Source: three-view drawing plus pictorial views. Frame: mm from the lowest corner of the part. Give positions to 0.01 mm unless a question says otherwise; leave off trailing zeros. Loops run counter-clockwise (first coordinate to the right, second up) from the corner with the lowest first, then second, coordinate; pieces in that order, holes last. Notation, with made-up numbers: (-8.75, 68.25) -> (25.25, 68.25) arc R18 ccw to (25.25, 90.25) -> close; hole circle Ø5 at (37, -26.75). An arc over 180 degrees is marked (long way). One line per item, written item: value. Start each with the question number.
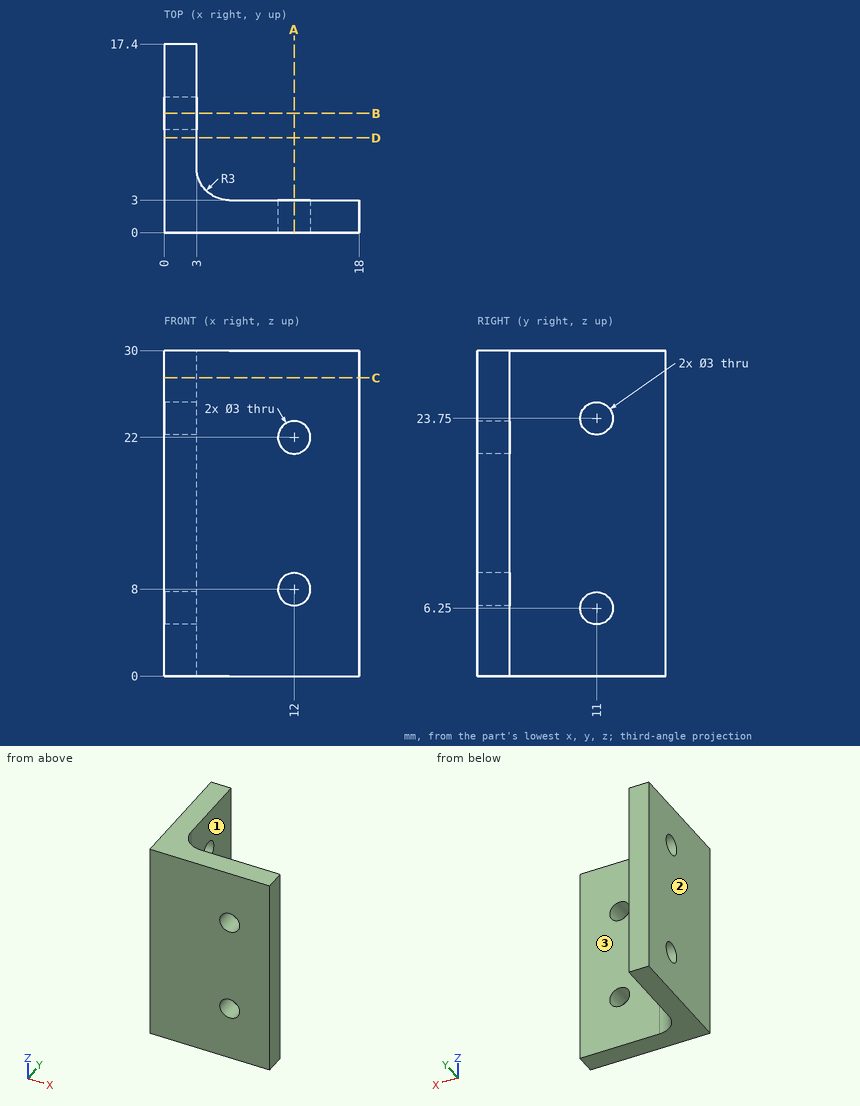
Item 1: Section A-A, the plane x = 12. Output: boundary loops of the cut face in (y, z), then the cut area to 3 significant figures.
Item 2: Ray query, line 1 along Z through (x, y) = (1, 11); line 2 along Y through (x, z) = (2.45, 23.75); line 3 along X through (y, z) = (2.35, 8). Return the intervals inside material, ascending. Write a range as [from, to].
Item 3: Pin query (flat end, axial travel): pin 1 (10 mm diameter, centred on y = 15.5, z = 23, fed in from +X); pin 2 (5 mm diameter, centred on x = 11, z = 18.5, fed in from +Y). Return the tip coordinate at first contact, or that it passes through.
Item 4: Section B-B, the plane y = 11. Output: boundary loops of the cut face in (x, z).
Item 5: Section C-C, the plane z = 27.5. Output: boundary loops of the cut face in (x, y), then the cut area to 3 significant figures.
Item 6: Mould query, pull axis X, two halves, no side actions, for the marked faces 1, 2 and 3. Classes: pulls with the +X half, pulls with the -X half, needs draft (parallel to the pull), parting line crosses it, or undercut.
Item 7: Section D-D, the plane y = 8.75. Output: boundary loops of the cut face in (x, z).
Geometry check:
1. outline: (0, 0) -> (3, 0) -> (3, 6.5) -> (0, 6.5) -> close; (0, 9.5) -> (3, 9.5) -> (3, 20.5) -> (0, 20.5) -> close; (0, 23.5) -> (3, 23.5) -> (3, 30) -> (0, 30) -> close
1. area: 72.0 mm2
2. line 1: z = [0, 4.75], [7.75, 22.25], [25.25, 30]
2. line 2: y = [0, 9.5], [12.5, 17.4]
2. line 3: x = [0, 10.5], [13.5, 18]
3. pin 1: stops at x = 3
3. pin 2: stops at y = 3
4. outline: (0, 0) -> (3, 0) -> (3, 4.75) -> (0, 4.75) -> close; (0, 7.75) -> (3, 7.75) -> (3, 22.25) -> (0, 22.25) -> close; (0, 25.25) -> (3, 25.25) -> (3, 30) -> (0, 30) -> close
5. outline: (0, 0) -> (18, 0) -> (18, 3) -> (6, 3) arc R3 cw to (3, 6) -> (3, 17.4) -> (0, 17.4) -> close
5. area: 99.1 mm2
6. face 1: pulls with the +X half
6. face 2: pulls with the -X half
6. face 3: needs draft
7. outline: (0, 0) -> (3, 0) -> (3, 30) -> (0, 30) -> close
